from build123d import *

# Parameters (mm, degrees)
SKETCH1_R               = 8.189006913
BOSS_EXTRUDE1_DEPTH     = 30
SKETCH2_R               = 3
CUT_EXTRUDE1_DEPTH      = 30
SKETCH4_W               = 1.839212521
SKETCH4_H               = 4.190652527
BOSS_EXTRUDE2_DEPTH     = 10
SKETCH3_R               = 1.5
CUT_EXTRUDE2_DEPTH      = 10
CUT_EXTRUDE2_DEPTH_BACK = 10


with BuildPart() as part:
    # Sketch1 → Boss-Extrude1 (new body)
    with BuildSketch(Plane(origin=(0, 0, 0), x_dir=(1, 0, 0), z_dir=(0, 1, 0))):
        Circle(SKETCH1_R)
    extrude(amount=BOSS_EXTRUDE1_DEPTH)

    # Sketch2 → Cut-Extrude1 (cut)
    with BuildSketch(Plane(origin=(0, 30, 0), x_dir=(1, 0, 0), z_dir=(0, 1, 0))):
        Circle(SKETCH2_R)
    extrude(amount=-CUT_EXTRUDE1_DEPTH, mode=Mode.SUBTRACT)

    # Sketch4 → Boss-Extrude2 (add)
    with BuildSketch(Plane(origin=(0, 30, 0), x_dir=(1, 0, 0), z_dir=(0, 1, 0))):
        with Locations((-3.214713917, 0.163363311)):
            Rectangle(SKETCH4_W, SKETCH4_H)
    extrude(amount=-BOSS_EXTRUDE2_DEPTH)

    # Sketch3 → Cut-Extrude2 (cut, two sides)
    with BuildSketch(Plane(origin=(0, 0, 0), x_dir=(0, 0, -1), z_dir=(1, 0, 0))) as cut_extrude2_sk:
        with Locations((0, 15)):
            Circle(SKETCH3_R)
    extrude(amount=CUT_EXTRUDE2_DEPTH, mode=Mode.SUBTRACT)
    extrude(cut_extrude2_sk.sketch, amount=-CUT_EXTRUDE2_DEPTH_BACK, mode=Mode.SUBTRACT)


solid = part.part
Read the model definition and answer for the solid it produces. Units are mm, in the model's axes. A direction names the side the tool comes from. Coordinates: 2 decimals unless noted, no trailing zeros. Write each loop counter-clockwise with the first axis right and the second up, starting at its lowest first coordinate (ties: lowest second). Pieces come first, ordered by that corner, then holes. Notation, with made-up numbers: (84.25, 46.5) - (141.25, 46.5) arc R19 ccw to (141.25, 66.5) - close; hole circle Ø1 at (-5.75, 18). An arc over 180 degrees is marked (long way). One line per question, with ' | ' between items.
Q1. Each of these flat-tipped pins is pushed along its axis until it touches: P1, Ø0.8, axis at x = -2.5, z = -0.5, coming from the -Y side; P2, Ø5, axis at y = 10, z = -3, coming from the -X side; P3, Ø5, axis at x = 5.5, z = -6, coming from the -Y side; P4, Ø6, axis at y = 26.5, z = -6, coming from the -X side. Where does it stop, or does it pass through?
Result set:
P1: y = 20 | P2: x = -8.17 | P3: y = 0 | P4: x = -7.62
Q2. Find section D-D, the plane x = -5.75. Write down the section's boundary in (y, z).
Result set:
outline: (0, -5.83) - (30, -5.83) - (30, 5.83) - (0, 5.83) - close; hole circle Ø3 at (15, 0)
Q3. Find section B-B, the plane z = 0. Write down the section's boundary in (x, y).
Result set:
outline: (-8.19, 0) - (-3, 0) - (-3, 13.5) - (-8.19, 13.5) - close; (-8.19, 16.5) - (-3, 16.5) - (-3, 20) - (-2.3, 20) - (-2.3, 30) - (-8.19, 30) - close; (3, 0) - (8.19, 0) - (8.19, 13.5) - (3, 13.5) - close; (3, 16.5) - (8.19, 16.5) - (8.19, 30) - (3, 30) - close
Q4. Determine the mould class of faces 3 (the flat face through (-2.295, 25, 0)), 4 (the cylindrical face through (-5.35, 15.07, 1.5)), 5 (the flat face through (4, 0, 0)), 6 (the cylindrical face through (7.8, 14.8, -2.5)) for opening direction Z: +Z half, -Z half, draft (parallel to the pull), parting line (faces both ways), or undercut.
Result set:
face 3: undercut | face 4: undercut | face 5: draft | face 6: parting line
Q5. Find section C-C, the plane y = 14. Write down the section's boundary in (x, z).
Result set:
outline: (-8.11, -1.12) arc R8.19 ccw to (8.11, -1.12) - (2.78, -1.12) arc R3 cw to (-2.78, -1.12) - close; (-8.11, 1.12) - (-2.78, 1.12) arc R3 cw to (2.78, 1.12) - (8.11, 1.12) arc R8.19 ccw to start
Q6. For faces 1 (the cylindrical face through (1.61, 15.21, -2.53)), 2 (the flat face through (4, 30, 0)), determine the directions among +Z, -Z, +X, -X, +Y, -Y from which every point of the face is accessible in a straight line to the end or side of a thin tool.
Result set:
face 1: -Y | face 2: +Z, -Z, +X, -X, +Y
Q7. Consider L1, parallel to Y at x = -4.95, z = 0; L2, parallel to Z at x = 0, y = 19.5; L3, parallel to Z at x = 4.15, y = 15. Determine where each line is inside the solid, lowest interval first. Write a range as [from, to].
Result set:
L1: [0, 13.5], [16.5, 30] | L2: [-8.19, -3], [3, 8.19] | L3: [-7.06, -1.5], [1.5, 7.06]
Q8. Find section A-A, the plane x = 0. Write down the section's boundary in (y, z), plus the area to 3 significant figures.
Result set:
outline: (0, -8.19) - (30, -8.19) - (30, -3) - (0, -3) - close; (0, 3) - (30, 3) - (30, 8.19) - (0, 8.19) - close | area: 311 mm^2
